```python
from build123d import *

# Parameters (mm, degrees)
F2_R     = 1.2
F3_SIZE2 = 0.2886751346
F3_SIZE  = 0.5
F4_R     = 1


with BuildPart() as f1:
    # F0 (on Front) → F1 (revolve)
    with BuildSketch(Plane.XZ):
        Polygon((-7.75, 0), (0, 0), (0, 12.2), (-1.9, 12.2), (-1.9, 2.2), (-4, 2.2), (-4, 1.5), (-7.75, 1.5), align=None)
    revolve(axis=Axis((0, 0, 5.0761818423), (0, 0, 1)))

    # F2
    f2_edges = [f1.edges().sort_by_distance(p)[0] for p in [
        (7.75, 0, 0),
    ]]
    fillet(f2_edges, radius=F2_R)

    # F3
    f3_edges = [f1.edges().sort_by_distance(p)[0] for p in [
        (1.9, 0, 12.2),
    ]]
    chamfer(f3_edges, length=F3_SIZE, length2=F3_SIZE2)

    # F4
    f4_edges = [f1.edges().sort_by_distance(p)[0] for p in [
        (1.9, 0, 11.7),
    ]]
    fillet(f4_edges, radius=F4_R)


solid = f1.part
```
The listing builds one solid part. Answer for the finished solid, in the listing's coordinates (mm). A direction names the side the tool comes from. Coordinates: 2 decimals unless noted, no trailing zeros. Loops run counter-clockwise (first coordinate to the right, second up) from the corner with the lowest first, then second, coordinate; pieces in that order, holes last. Notation, with made-up numbers: (25.5, -37) -> (45.5, -37) arc R32 cw to (45.5, -9) -> close; hole circle Ø6 at (-23, -22). An arc over 180 degrees is marked (long way). Return JSON: item names as keys, results as strings. Group by question number.
(1) Find the intervals of material crossed by probe 1 along Z at (x, y) = (1.25, -3.75); probe 2 along Y at (x, z) = (0, 7.5); probe 3 along Z at (x, y) = (1, 4.25), in increasing order. Write a range as from..to.
(2) Which of the six approach directions +Z, -Z, +X, -X, +Y, -Y give full straight-line access (tool end or side, diameter ignored) to faces 1 (the cylindrical face through (1.9, -0.08, 6.75)), 2 (the flat face through (0, 0, 0))?
(3) Given pin 1 Ø1 at (y, z) = (0.5, 9.5) entering from +X; pin 2 Ø1 at (x, z) = (0, 2.5) entering from -Y, each flat-ended and moving along its own axis, determine where each tip first touches the part or whether it passes through.
(4) A cutting plane is placed at A-A on z = 5. Write down the section's boundary in (x, y), and give its area (3 significant figures).
The answers:
{
 "1": {"probe 1": "z = 0..2.2", "probe 2": "y = -1.9..1.9", "probe 3": "z = 0..1.5"},
 "2": {"face 1": "+Z", "face 2": "-Z, +X, -X, +Y, -Y"},
 "3": {"pin 1": "stops at x = 1.9", "pin 2": "stops at y = -4"},
 "4": {"outline": "circle Ø3.8 at (0, 0)", "area": "11.3 mm^2"}
}
